Geometry: final body of the model. Coordinates: model frame, mm. A direction names the side the tool comes from. Give positions to 0.01 mm unless a question says otherwise; leave off trailing zeros. Write each loop counter-clockwise with the first axis right and the second up, starting at its lowest first coordinate (ties: lowest second). Pieces come first, ordered by that corner, then holes. Notation, with made-up numbers: (16, -13.5) - (37, -13.5) arc R18 ccw to (37, -7.5) - close; hole circle Ø8 at (-0.5, 12.5). An arc over 180 degrees is marked (long way). Return JSON: item names as keys, results as strings.
from build123d import *

# Parameters (mm, degrees)
F1_DEPTH = 20
F2_R     = 2.65
F3_DEPTH = 20.001
F4_R     = 1.6
F5_DEPTH = 7.001
F6_R     = 2
F7_R     = 1


with BuildPart() as f1:
    # F0 (on Front) → F1 (new body)
    with BuildSketch(Plane.XZ):
        with BuildLine():
            Line((3.5, -10), (3.5, 0))
            ThreePointArc((3.5, 0), (0, 3.5), (-3.5, 0))
            Line((-3.5, 0), (-3.5, -10))
            Line((-3.5, -10), (3.5, -10))
        make_face()
    extrude(amount=F1_DEPTH)

    # F2 (on face) → F3 (cut, through all)
    with BuildSketch(Plane(origin=(0, 0, 0), x_dir=(-1, 0, 0), z_dir=(0, 1, 0))):
        Circle(F2_R)
        with BuildLine():
            ThreePointArc((2, -3.464102), (0, -4), (-2, -3.464102))
            Line((-2, -3.464102), (-2, -8.5))
            Line((-2, -8.5), (2, -8.5))
            Line((2, -8.5), (2, -3.464102))
        make_face()
    extrude(amount=-F3_DEPTH, mode=Mode.SUBTRACT)

    # F4 (on face) → F5 (cut, through all)
    with BuildSketch(Plane(origin=(-3.5, 0, 0), x_dir=(0, -1, 0), z_dir=(-1, 0, 0))):
        with Locations((5.2, -4.5)):
            Circle(F4_R)
    extrude(amount=-F5_DEPTH, mode=Mode.SUBTRACT)

    # F6
    f6_edges = [f1.edges().sort_by_distance(p)[0] for p in [
        (-3.5, -10, -10),
        (3.5, -10, -10),
    ]]
    fillet(f6_edges, radius=F6_R)

    # F7
    f7_edges = [f1.edges().sort_by_distance(p)[0] for p in [
        (2, -10, -8.5),
        (-2, -10, -8.5),
    ]]
    fillet(f7_edges, radius=F7_R)


solid = f1.part
Q1. Section query D-D, the plane x = 0. Return the cut outline in (y, z), plus the area to 3 significant figures.
Answer key:
{"outline": "(-20, -10) - (0, -10) - (0, -8.5) - (-20, -8.5) - close; (-20, -4) - (-6.72, -4) arc R1.6 cw to (-3.68, -4) - (0, -4) - (0, -2.65) - (-20, -2.65) - close; (-20, 2.65) - (0, 2.65) - (0, 3.5) - (-20, 3.5) - close", "area": "71.6 mm^2"}
Q2. Pin query (flat end, axial travel): P1, Ø5, axis at y = -5.2, z = -4.5, coming from the -X side; P2, Ø1, axis at x = 2.5, y = -8, coming from the +Z side. Return the tip coordinate at first contact, or that it passes through.
Answer key:
{"P1": "stops at x = -3.5", "P2": "stops at z = 2.87"}
Q3. Mould query, pull axis Y, two halves, no side actions, for faces 3 (the cylindrical face through (-0.049, -4.992, -2.914)), 4 (the cylindrical face through (-2.45, -9.86, -1.01)), 5 (the flat face through (0, -20, -3)). Classes: pulls with the +Y half, pulls with the -Y half, needs draft (parallel to the pull), parting line crosses it, or undercut.
Answer key:
{"face 3": "undercut", "face 4": "needs draft", "face 5": "pulls with the -Y half"}
Q4. Section query A-A, the plane y = -5.2. Return the cut outline in (x, z), plus the area to 3 significant figures.
Answer key:
{"outline": "(-3.5, -8) arc R2 ccw to (-1.5, -10) - (1.5, -10) arc R2 ccw to (3.5, -8) - (3.5, -6.1) - (2, -6.1) - (2, -7.5) arc R1 cw to (1, -8.5) - (-1, -8.5) arc R1 cw to (-2, -7.5) - (-2, -6.1) - (-3.5, -6.1) - close; (-3.5, -2.9) - (3.5, -2.9) - (3.5, 0) arc R3.5 ccw to (-3.5, 0) - close; hole circle Ø5.3 at (0, 0)", "area": "33.9 mm^2"}
Q5. Section query B-B, the plane z = -6.5. Return the cut outline in (x, y), plus the area to 3 significant figures.
Answer key:
{"outline": "(-3.5, -20) - (-2, -20) - (-2, 0) - (-3.5, 0) - close; (2, -20) - (3.5, -20) - (3.5, 0) - (2, 0) - close", "area": "60.0 mm^2"}
Q6. Material intervals for probe 1 along Z at (x, y) = (0, -14.5); probe 2 along X at (y, z) = (-15.5, -6.75); probe 3 along Z at (x, y) = (0.25, -5.2), sorted ascending. Write a range as [from, to].
Answer key:
{"probe 1": "z = [-10, -8.5], [-4, -2.65], [2.65, 3.5]", "probe 2": "x = [-3.5, -2], [2, 3.5]", "probe 3": "z = [-10, -8.5], [-2.9, -2.64], [2.64, 3.49]"}
Q7. Set-up query: faces 1 (the flat face through (3.5, -10, -4)), 2 (the cylindrical face through (-1.715, -10.14, -8.199)). Return all of +Z, -Z, +X, -X, +Y, -Y with unobstructed straight access to the full face (end or side cutting, diameter ignored); none if empty.
Answer key:
{"face 1": "+Z, -Z, +X, +Y, -Y", "face 2": "+Y, -Y"}
Q8. Section query C-C, the plane y = -8. Return the cut outline in (x, z).
Answer key:
{"outline": "(-3.5, -8) arc R2 ccw to (-1.5, -10) - (1.5, -10) arc R2 ccw to (3.5, -8) - (3.5, 0) arc R3.5 ccw to (-3.5, 0) - close; hole circle Ø5.3 at (0, 0); hole (-2, -7.5) arc R1 ccw to (-1, -8.5) - (1, -8.5) arc R1 ccw to (2, -7.5) - (2, -3.46) arc R4 cw to (-2, -3.46) - close"}
